from build123d import *

# Parameters (mm, degrees)
BOSS_EXTRUDE2_DEPTH = 10
FILLET1_R           = 5
SKETCH7_W           = 380
SKETCH7_H           = 53
SKETCH7_W_2         = 80
SKETCH7_H_2         = 170
CUT_EXTRUDE1_DEPTH  = 10


with BuildPart() as part:
    # Sketch1 → Boss-Extrude2 (new body)
    with BuildSketch(Plane(origin=(0, 0, 0), x_dir=(1, 0, 0), z_dir=(0, 1, 0))):
        Polygon((-300, 105), (-250, 155), (300, 155), (300, -155), (-250, -155), (-300, -105), align=None)
    extrude(amount=BOSS_EXTRUDE2_DEPTH)

    # Fillet1
    fillet1_edges = [part.edges().sort_by_distance(p)[0] for p in [
        (300, 5, 155),
        (-250, 5, 155),
        (-300, 5, 105),
        (-300, 5, -105),
        (-250, 5, -155),
        (300, 5, -155),
        (-275, 10, -130),
        (-300, 10, 0),
        (-275, 10, 130),
        (25, 10, 155),
        (300, 10, 0),
        (25, 10, -155),
    ]]
    fillet(fillet1_edges, radius=FILLET1_R)

    # Sketch7 → Cut-Extrude1 (cut)
    with BuildSketch(Plane.XZ):
        with Locations((-10, -122.5)):
            Rectangle(SKETCH7_W, SKETCH7_H)
        with Locations((-10, 122.5)):
            Rectangle(SKETCH7_W, SKETCH7_H)
        with Locations((-150, 0)):
            Rectangle(SKETCH7_W_2, SKETCH7_H_2)
    extrude(amount=-CUT_EXTRUDE1_DEPTH, mode=Mode.SUBTRACT)


solid = part.part
Source: CAD feature listing. Evaluate the final solid. Frame: model axes, mm. Give positions to 0.01 mm unless a question says otherwise; leave off trailing zeros. Write each loop counter-clockwise with the first axis right and the second up, starting at its lowest first coordinate (ties: lowest second). Pieces come first, ordered by that corner, then holes. Notation, with made-up numbers: M -28.5,-14.75 L 28.5,-14.75 A19 ccw 28.5,4.25 Z; hole C 46,88 d11. An arc over 180 degrees is marked long. Return JSON: item names as keys, results as strings. Group by question number.
1) Cut plane D-D, the plane x = 81. Output: boundary loops of the cut face in (y, z), plus the area to 3 significant figures.
2) Pin query (flat end, axial travel): P1, Ø1.5, axis at y = 6.5, z = -40.5, coming from the +X side; P2, Ø1, axis at y = 6, z = -70.5, coming from the +X side. Return the tip coordinate at first contact, or that it passes through.
3) Material intervals for line 1 along Z through (x, y) = (85.5, 4); line 2 along Z through (x, y) = (-174, 5.25); line 3 along X through (y, z) = (3, 17), sorted ascending. Write a range as [from, to].
4) Cut plane A-A, the plane z = -7. Output: boundary loops of the cut face in (x, y), plus the area to 3 significant figures.
5) Cut plane C-C, the plane y = 3.5. Output: boundary loops of the cut face in (x, z), plus the area to 3 significant figures.
6) Cut plane B-B, the plane x = -144.5. Output: boundary loops of the cut face in (y, z).
Recorded:
{
 "1": {"outline": "M 0,-155 L 5,-155 A5 ccw 10,-150 L 10,-149 L 0,-149 Z; M 0,-96 L 10,-96 L 10,96 L 0,96 Z; M 0,149 L 10,149 L 10,150 A5 ccw 5,155 L 0,155 Z", "area": "2,030 mm²"},
 "2": {"P1": "stops at x = 299.94", "P2": "stops at x = 299.97"},
 "3": {"line 1": "z = [-155, -149], [-96, 96], [149, 155]", "line 2": "z = [-154.99, -149], [-96, -85], [85, 96], [149, 154.99]", "line 3": "x = [-300, -190], [-110, 300]"},
 "4": {"outline": "M -300,0 L -190,0 L -190,10 L -295,10 A5 ccw -300,5 Z; M -110,0 L 300,0 L 300,5 A5 ccw 295,10 L -110,10 Z", "area": "5,190 mm²"},
 "5": {"outline": "M -300,-102.93 A5 ccw -298.54,-106.46 L -251.46,-153.54 A5 ccw -247.93,-155 L 295,-155 A5 ccw 300,-150 L 300,150 A5 ccw 295,155 L -247.93,155 A5 ccw -251.46,153.54 L -298.54,106.46 A5 ccw -300,102.93 Z; hole M -200,-149 L 180,-149 L 180,-96 L -200,-96 Z; hole M -200,96 L 180,96 L 180,149 L -200,149 Z; hole M -190,-85 L -110,-85 L -110,85 L -190,85 Z", "area": "130,000 mm²"},
 "6": {"outline": "M 0,-155 L 5,-155 A5 ccw 10,-150 L 10,-149 L 0,-149 Z; M 0,-96 L 10,-96 L 10,-85 L 0,-85 Z; M 0,85 L 10,85 L 10,96 L 0,96 Z; M 0,149 L 10,149 L 10,150 A5 ccw 5,155 L 0,155 Z"}
}
